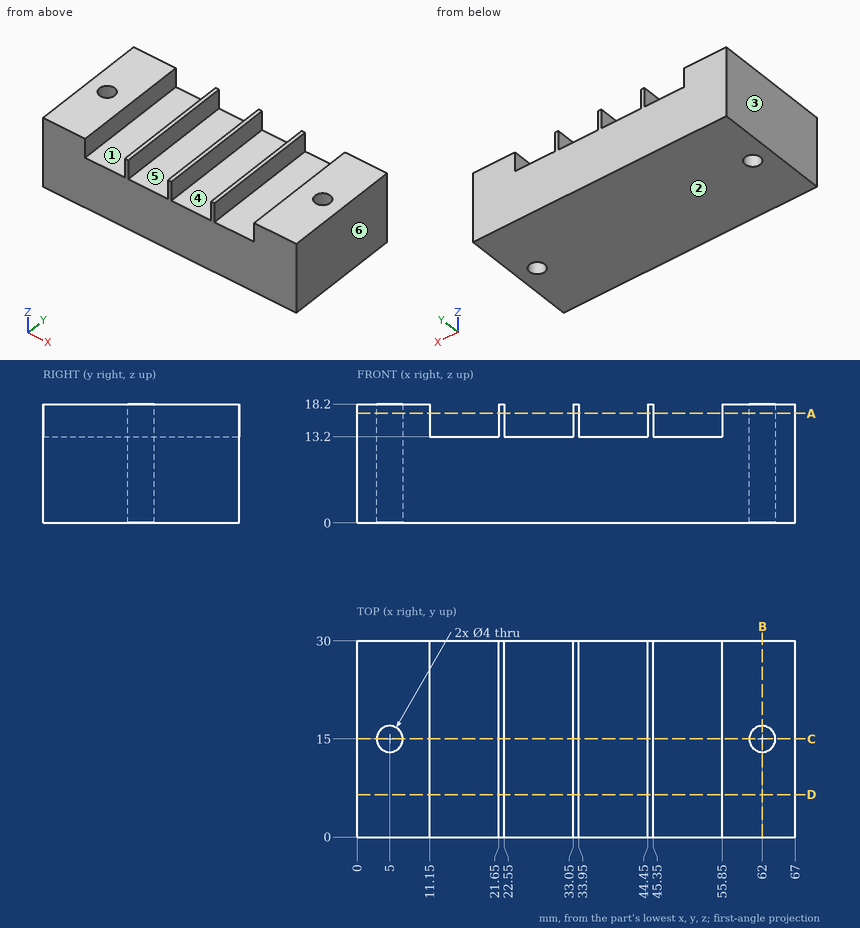
Check sheet for the drawn part. Datum: minimum x, y, z corner. Units: mm. A direction names the side the tool comes from. Coordinates: 2 decimals unless noted, no trailing zeros. Write each loop counter-clockwise with the first axis right and the second up, starting at its lowest first coordinate (ties: lowest second). Pieces come first, ordered by that corner, then holes. Notation, with made-up numbers: M -31,-4 L 1,-4 A28 cw 1,16 Z; hole C -14.75,2.25 d2. An arc over 180 degrees is marked long. Use a Markdown table: item, result.
Q1. Sectioned sample at D-D, the plane y = 6.5. Record the boundary of the cut face in (x, z), plus the area to 3 significant figures.
Reply:
| item | result |
|---|---|
| outline | M 0,0 L 67,0 L 67,18.2 L 55.85,18.2 L 55.85,13.2 L 45.35,13.2 L 45.35,18.2 L 44.45,18.2 L 44.45,13.2 L 33.95,13.2 L 33.95,18.2 L 33.05,18.2 L 33.05,13.2 L 22.55,13.2 L 22.55,18.2 L 21.65,18.2 L 21.65,13.2 L 11.15,13.2 L 11.15,18.2 L 0,18.2 Z |
| area | 1,010 mm² |
Q2. Sectioned sample at C-C, the plane y = 15. Record the boundary of the cut face in (x, z), plus the area to 3 significant figures.
Reply:
| item | result |
|---|---|
| outline | M 0,0 L 3,0 L 3,18.2 L 0,18.2 Z; M 7,0 L 60,0 L 60,18.2 L 55.85,18.2 L 55.85,13.2 L 45.35,13.2 L 45.35,18.2 L 44.45,18.2 L 44.45,13.2 L 33.95,13.2 L 33.95,18.2 L 33.05,18.2 L 33.05,13.2 L 22.55,13.2 L 22.55,18.2 L 21.65,18.2 L 21.65,13.2 L 11.15,13.2 L 11.15,18.2 L 7,18.2 Z; M 64,0 L 67,0 L 67,18.2 L 64,18.2 Z |
| area | 864 mm² |
Q3. Set-up check for the marked faces 1 and 2: record each of +Z, -Z, +X, -X, +Y, -Y from which the full face is reachable in a straight line by a thin tool's end or side.
Reply:
| item | result |
|---|---|
| face 1 | +Z, +Y, -Y |
| face 2 | -Z, +X, -X, +Y, -Y |
Q4. Draft check along X on the marked faces 3, 4, 5 and 6. Enter one of: +X half, -X half, draft (parallel to the pull), parting line (faces both ways), or undercut.
Reply:
| item | result |
|---|---|
| face 3 | -X half |
| face 4 | undercut |
| face 5 | undercut |
| face 6 | +X half |
Q5. Sectioned sample at A-A, the plane z = 16.75. Record the boundary of the cut face in (x, y), plus the area to 3 significant figures.
Reply:
| item | result |
|---|---|
| outline | M 0,0 L 11.15,0 L 11.15,30 L 0,30 Z; M 21.65,0 L 22.55,0 L 22.55,30 L 21.65,30 Z; M 33.05,0 L 33.95,0 L 33.95,30 L 33.05,30 Z; M 44.45,0 L 45.35,0 L 45.35,30 L 44.45,30 Z; M 55.85,0 L 67,0 L 67,30 L 55.85,30 Z; hole C 5,15 d4; hole C 62,15 d4 |
| area | 725 mm² |
Q6. Thickness scan on line 1 (X direction, y = 18.75, z = 16.5); line 2 (Y direction, x = 5, z = 10); line 3 (X direction, y = 16, z = 8.5). Record the ranges inside material, lowest first.
Reply:
| item | result |
|---|---|
| line 1 | x = 0 to 11.15, 21.65 to 22.55, 33.05 to 33.95, 44.45 to 45.35, 55.85 to 67 |
| line 2 | y = 0 to 13, 17 to 30 |
| line 3 | x = 0 to 3.27, 6.73 to 60.27, 63.73 to 67 |
Q7. Sectioned sample at B-B, the plane x = 62. Record the boundary of the cut face in (y, z), plus the area to 3 significant figures.
Reply:
| item | result |
|---|---|
| outline | M 0,0 L 13,0 L 13,18.2 L 0,18.2 Z; M 17,0 L 30,0 L 30,18.2 L 17,18.2 Z |
| area | 473 mm² |
Q8. Go/stop test with a flat-tipped pin: P1, Ø5, axis at x = 38, y = 17, coming from the +Z side. Record where the tip stops, or that it passes through.
Reply:
| item | result |
|---|---|
| P1 | stops at z = 13.2 |
